For this review, use the dimensioned drawing (mm, ordinates from the lowest corner) and the shaded views. A direction names the side the tool comes from. Round coordinates to 2 decimals unless told otherwise and drop trailing zeros. Order: outer loops, then holes, each group sorted by start corner. A loop starts at its lowest first (then second) coordinate and runs counter-clockwise, first axis right, second up. Notation, with made-up numbers: (43, 70) - (62, 70) arc R25 cw to (62, 97) - close; hole circle Ø8 at (-33.75, 64.5). An arc over 180 degrees is marked (long way). Use CSV: the item, a comma, the result in double quotes. Start each with the question number.
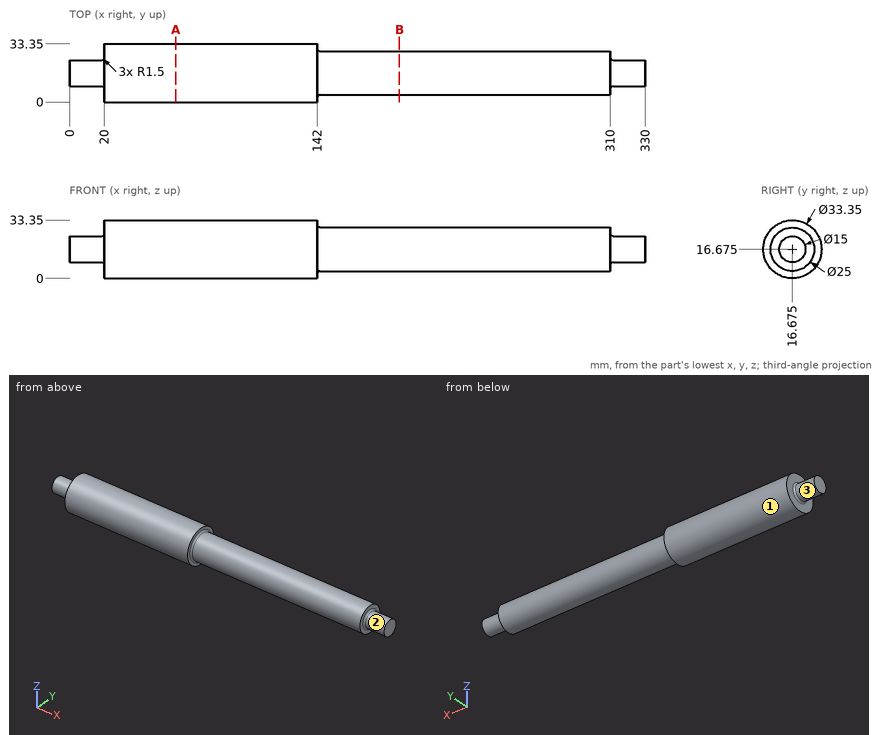
Q1. For L1, parallel to X at y = 8.5, z = 22; L2, parallel to X at y = 1.5, z = 18.5; L3, parallel to Y at x = 266, z = 17.5, list the stretches that pass through material, from the lowest coordinate up. Write a range as [from, to].
Q2. Take a section at B-B (x = 189). State the section outline as (y, z) points (3 decimals), plus the area to 3 significant figures.
Q3. Clearance check with flat-ended pins moving along their axes: pin 1 (6 mm diameter, centred on x = 40.5, z = 28.5, fed in from +Y); pin 2 (1 mm diameter, centred on x = 277, z = 23.5, fed in from -Y); pin 3 (12 mm diameter, centred on x = 161.5, y = 7, fed in from +Z). State where each tip first meets the part, or that it passes through.
Q4. Take a section at A-A (x = 61). State the section outline as (y, z) points (3 decimals), plus the area to 3 significant figures.
Q5. Tool access review of the marked faces 1, 2 and 3: name each direction out of +Z, -Z, +X, -X, +Y, -Y from which nothing blocks a thin tool from reaching the whole face with its end or side.
Findings below:
1,L1,"x = [20, 310]"
1,L2,"x = [20, 142]"
1,L3,"y = [4.2, 29.15]"
2,outline,"circle Ø25 at (16.675, 16.675)"
2,area,"491 mm^2"
3,pin 1,"stops at y = 30.82"
3,pin 2,"stops at y = 5.89"
3,pin 3,"stops at z = 28.62"
4,outline,"circle Ø33.35 at (16.675, 16.675)"
4,area,"874 mm^2"
5,face 1,"+X, -X"
5,face 2,"+X"
5,face 3,"-X"
